Here's how the part is built. I have some questions about the finished solid (model axes, mm). A direction names the side the tool comes from. Coordinates: 2 decimals unless noted, no trailing zeros. Loops run counter-clockwise (first coordinate to the right, second up) from the corner with the lowest first, then second, coordinate; pieces in that order, holes last. Notation, with made-up numbers: (-2, -23.75) - (13, -23.75) arc R11 cw to (13, -7.75) - close; hole circle Ø2 at (-28, -10). An arc over 180 degrees is marked (long way). Use a Markdown table: item, result.
```python
from build123d import *

# Parameters (mm, degrees)
SKETCH_1_R            = 5.6
EXTRUDE_394_DEPTH     = 10
SKETCH_3_R            = 1.2
CUT_EXTRUDE_678_DEPTH = 11


with BuildPart() as part:
    # Эскиз1 → Extrude 394 (new, symmetric)
    with BuildSketch(Plane.XY):
        with BuildLine():
            Line((-10.6, 0), (-10.6, -10.6))
            Line((-10.6, -10.6), (10.6, -10.6))
            Line((10.6, -10.6), (10.6, 0))
            ThreePointArc((10.6, 0), (0, 10.6), (-10.6, 0))
        make_face()
        Circle(SKETCH_1_R, mode=Mode.SUBTRACT)
    extrude(amount=EXTRUDE_394_DEPTH, both=True)

    # Эскиз3 → Cut-Extrude 678 (cut)
    with BuildSketch(Plane.XZ.offset(10.6)):
        with Locations(Location((-7.5, 0, 0), (0, 0, 270))):
            Circle(SKETCH_3_R)
        with Locations(Location((7.5, 0, 0), (0, 0, 90))):
            Circle(SKETCH_3_R)
    extrude(amount=-CUT_EXTRUDE_678_DEPTH, mode=Mode.SUBTRACT)


solid = part.part
```
Q1. Will these pins go through, and if not, where does the flat tip stop? P1, Ø6, axis at x = -7, z = -7, coming from the +Y side; P2, Ø1.9, axis at x = 7.5, z = 0, coming from the -Y side; P3, Ø8, axis at x = -5, y = 2, coming from the -Z side; P4, Ø2, axis at x = -7.5, z = 0, coming from the +Y side.
Check values:
| item | result |
|---|---|
| P1 | y = 9.82 |
| P2 | y = 0.4 |
| P3 | z = -10 |
| P4 | y = 8.37 |
Q2. I want a section at B-B, the plane y = -5.25. Write out the boundary of the cut face in (x, z), then the cut area to 3 significant figures.
Check values:
| item | result |
|---|---|
| outline | (-10.6, -10) - (-1.95, -10) - (-1.95, 10) - (-10.6, 10) - close; (1.95, -10) - (10.6, -10) - (10.6, 10) - (1.95, 10) - close; hole circle Ø2.4 at (-7.5, 0); hole circle Ø2.4 at (7.5, 0) |
| area | 337 mm^2 |
Q3. Please list where these lines run through material, in increasing order: L1, parallel to X at y = -6, z = 0; L2, parallel to X at y = -2.5, z = 0; L3, parallel to Y at x = 3.25, z = -7. Write a range as from..to.
Check values:
| item | result |
|---|---|
| L1 | -10.6..-8.7, -6.3..6.3, 8.7..10.6 |
| L2 | -10.6..-8.7, -6.3..-5.01, 5.01..6.3, 8.7..10.6 |
| L3 | -10.6..-4.56, 4.56..10.09 |
Q4. I want a section at C-C, the plane y = -8.25. Write out the boundary of the cut face in (x, z), then the cut area to 3 significant figures.
Check values:
| item | result |
|---|---|
| outline | (-10.6, -10) - (10.6, -10) - (10.6, 10) - (-10.6, 10) - close; hole circle Ø2.4 at (-7.5, 0); hole circle Ø2.4 at (7.5, 0) |
| area | 415 mm^2 |
Q5. Which directions (+Z, -Z, +X, -X, +Y, -Y) give clear straight access to the entire face, cutting with the end or side of a thin tool? Please do faces 4 (the face through (-5.595, 0.246, -0.14)), 5 (the face through (6.31, -5.18, -0.16)).
Check values:
| item | result |
|---|---|
| face 4 | +Z, -Z |
| face 5 | -Y |
Q6. If we mould it in two halves opening along Z, with no side actions, what happens to faces 1 (the face through (7, 0.4, 0)), 2 (the face through (0.2, 10.6, 0.1)), 3 (the face through (5, -5, 10))? For each: pulls with the +Z half, pulls with the -Z half, needs draft (parallel to the pull), parting line crosses it, or undercut.
Check values:
| item | result |
|---|---|
| face 1 | undercut |
| face 2 | needs draft |
| face 3 | pulls with the +Z half |
Q7. I want a section at D-D, the plane x = 4.25. Write out the boundary of the cut face in (y, z).
Check values:
| item | result |
|---|---|
| outline | (-10.6, -10) - (-3.65, -10) - (-3.65, 10) - (-10.6, 10) - close; (3.65, -10) - (9.71, -10) - (9.71, 10) - (3.65, 10) - close |
Q8. I want a section at A-A, the plane z = 0. Write out the boundary of the cut face in (x, y), then the cut area to 3 significant figures.
Check values:
| item | result |
|---|---|
| outline | (-10.6, -10.6) - (-8.7, -10.6) - (-8.7, 0.4) - (-6.3, 0.4) - (-6.3, -10.6) - (6.3, -10.6) - (6.3, 0.4) - (8.7, 0.4) - (8.7, -10.6) - (10.6, -10.6) - (10.6, 0) arc R10.6 ccw to (-10.6, 0) - close; hole circle Ø11.2 at (0, 0) |
| area | 250 mm^2 |
